Part model, mm, in its own coordinate system. Face numbers are marked on the shaded views. A direction names the side the tool comes from. Coordinates: 2 decimals unless noted, no trailing zeros. Write each loop counter-clockwise with the first axis right and the second up, starting at its lowest first coordinate (ties: lowest second). Pieces come first, ordered by that corner, then holes. Notation, with made-up numbers: M 81,18.25 L 87,18.25 A21 ccw 87,44.25 Z; hole C 64.25,31.25 d6. An arc over 180 degrees is marked long. Use a Markdown table: item, result. Add a question column.
Q1. Wall check: L1, parallel to X at y = 2.1, z = -0.25; L2, parallel to Z at x = 0.5, y = 1; L3, parallel to X at y = 0.6, z = 4. Give the ranges that are in metal, low to high. Write a range as from..to.
Q2. Tool access for the marked faces 4 and 5: list every direction of +Z, -Z, +X, -X, +Y, -Y with a clear straight run to the whole face (end or side of a thin tool).
Q3. Mould opens along Z. For the marked faces 1, 2 and 3 say: released by +Z, released by -Z, zero draft, split by the parting line, or undercut.
Q4. Slice it at A-A on y = 0.75. Write the cut outline in (x, z) (3 decimals).
Q5. Slice it at B-B on z = 7. Write the cut outline in (x, y), then the cut area to 3 significant figures.
Q6. Slice it at C-C on x = -1.25. Write the cut outline in (y, z), then the cut area to 3 significant figures.
Autodesk Inventor part; units mm, degrees
ref_plane "YZ Plane" through (0, 0, 0) normal (1, 0, 0) x (0, 1, 0)
ref_plane "XZ Plane" through (0, 0, 0) normal (0, 1, 0) x (-1, 0, 0)
ref_plane "XY Plane" through (0, 0, 0) normal (0, 0, 1) x (1, 0, 0)
sketch "Sketch1" plane through (0, 0, 0) normal (0, 1, 0) x (-1, 0, 0)
  circle A0 centre (0, 0) radius 9.525
  line L0 (0, -7.3152) -> (-6.3351, -3.6576)
  line L1 (-6.3351, -3.6576) -> (-6.3351, 3.6576)
  line L2 (-6.3351, 3.6576) -> (0, 7.3152)
  line L3 (0, 7.3152) -> (6.3351, 3.6576)
  line L4 (6.3351, 3.6576) -> (6.3351, -3.6576)
  line L5 (6.3351, -3.6576) -> (0, -7.3152)
  dimension "d0" = 19.05
  dimension "d1" = 7.3152
extrude "Extrusion1" add sketch "Sketch1" along normal blind 3.81
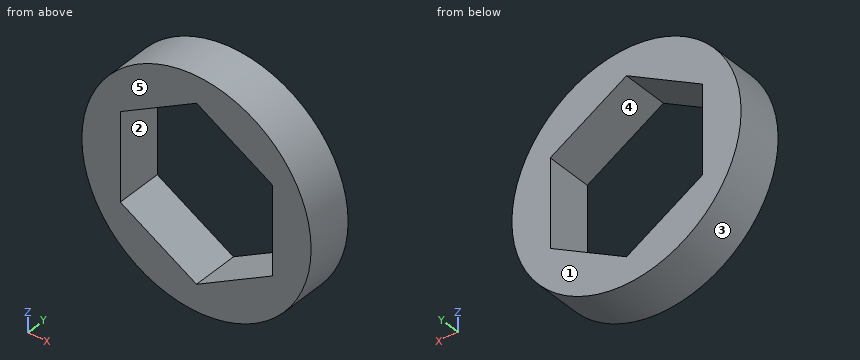
Recorded:
| question | item | result |
|---|---|---|
| 1 | L1 | -9.52..-6.34, 6.34..9.52 |
| 1 | L2 | -9.51..-7.03, 7.03..9.51 |
| 1 | L3 | -8.64..-5.74, 5.74..8.64 |
| 2 | face 4 | +Y, -Y |
| 2 | face 5 | +Z, -Z, +X, -X, -Y |
| 3 | face 1 | zero draft |
| 3 | face 2 | undercut |
| 3 | face 3 | split by the parting line |
| 4 | outline | C 0,0 d19.05; hole M -6.335,-3.658 L 0,-7.315 L 6.335,-3.658 L 6.335,3.658 L 0,7.315 L -6.335,3.658 Z |
| 5 | outline | M -6.46,0 L -0.55,0 L -0.55,3.81 L -6.46,3.81 Z; M 0.55,0 L 6.46,0 L 6.46,3.81 L 0.55,3.81 Z |
| 5 | area | 45.1 mm² |
| 6 | outline | M 0,-9.44 L 3.81,-9.44 L 3.81,-6.59 L 0,-6.59 Z; M 0,6.59 L 3.81,6.59 L 3.81,9.44 L 0,9.44 Z |
| 6 | area | 21.7 mm² |
